Here's how the part is built. I have some questions about the finished solid (model axes, mm). A direction names the side the tool comes from. Round coordinates to 2 decimals unless told otherwise and drop trailing zeros. Order: outer loops, then holes, each group sorted by start corner. A loop starts at its lowest first (then second) coordinate and runs counter-clockwise, first axis right, second up. Notation, with made-up numbers: (54.25, 20.5) -> (75.25, 20.5) arc R33 cw to (75.25, 59.5) -> close; hole circle Ø11 at (11, -6.5). An arc over 180 degrees is marked (long way). Use a Markdown table: item, result. Add a question column.
(1) I want a section at B-B, the plane x = -7.5. Please give me the cut outline in (y, z), then the cut area to 3 significant figures.
(2) I'm going to push flat-ended pins straight in: P1, Ø2.5, axis at x = -27, y = 0, coming from the +Z side; P2, Ø1.3, axis at x = 27, y = 0, coming from the -Z side; P3, Ø0.5, axis at y = -1.5, z = 0.5, coming from the -X side. Where does each tip first touch, or does it pass through?
(3) I want a section at C-C, the plane z = 0.6. Please give me the cut outline in (x, y).
(4) I want a section at A-A, the plane y = 0. Please give me the cut outline in (x, z), then the cut area to 3 significant figures.
(5) Thinking about a two-plate mould opening in Y: for faces 1 (the face through (-0.6, 4.05, 0.5)), 2 (the face through (-29.95, 0.13, 0.49)), 3 (the face through (0.3, 5.95, 0.5)), 4 (the face through (-26.237, 0.24, 0.507)), which applies, pulls with the +Y half, pulls with the -Y half, needs draft (parallel to the pull), parting line crosses it, or undercut?
(6) If I drill on probe 1 along Y at (x, z) = (-2.5, 0.9); probe 2 along X at (y, z) = (-0.25, 0.7); probe 3 along X at (y, z) = (0.5, 0.15), over which ranges is the centre line in solid material (lowest first)?
(7) On a 3-axis mill with a long thin cutter (end or side, diameter ignored), from which of +Z, -Z, +X, -X, +Y, -Y can I reach the whole of each face in a straight line? I mean faces 5 (the face through (-0.6, -4.15, 0.5)), 6 (the face through (0, 5, 1)). Say none if no direction works.
(8) I want a section at D-D, the plane x = 27. Please give me the cut outline in (y, z), then the cut area to 3 significant figures.
from build123d import *

# Parameters (mm, degrees)
BOSS_EXTRUDE2_DEPTH = 1
SKETCH4_R           = 0.8
CUT_EXTRUDE1_DEPTH  = 31.551677532
SKETCH5_W           = 15.2
SKETCH5_H           = 8.2
CUT_EXTRUDE2_DEPTH  = 31.551677532


with BuildPart() as part:
    # Sketch3 → Boss-Extrude2 (new body)
    with BuildSketch(Plane.XY):
        with BuildLine():
            Line((24, 5.95), (-24, 5.95))
            ThreePointArc((-24, 5.95), (-29.95, 0), (-24, -5.95))
            Line((-24, -5.95), (24, -5.95))
            ThreePointArc((24, -5.95), (29.95, 0), (24, 5.95))
        make_face()
    extrude(amount=BOSS_EXTRUDE2_DEPTH)

    # Sketch4 → Cut-Extrude1 (cut, through all)
    with BuildSketch(Plane.XY.offset(1)):
        with Locations((-27, 0)):
            Circle(SKETCH4_R)
        with Locations((27, 0)):
            Circle(SKETCH4_R)
    extrude(amount=-CUT_EXTRUDE1_DEPTH, mode=Mode.SUBTRACT)

    # Sketch5 → Cut-Extrude2 (cut, through all)
    with BuildSketch(Plane.XY.offset(1)):
        with Locations((-0.5, -0.05)):
            Rectangle(SKETCH5_W, SKETCH5_H)
    extrude(amount=-CUT_EXTRUDE2_DEPTH, mode=Mode.SUBTRACT)


solid = part.part
Taken from the geometry:
| question | item | result |
|---|---|---|
| 1 | outline | (-5.95, 0) -> (-4.15, 0) -> (-4.15, 1) -> (-5.95, 1) -> close; (4.05, 0) -> (5.95, 0) -> (5.95, 1) -> (4.05, 1) -> close |
| 1 | area | 3.70 mm2 |
| 2 | P1 | stops at z = 1 |
| 2 | P2 | passes through |
| 2 | P3 | stops at x = -29.82 |
| 3 | outline | (-24, -5.95) -> (24, -5.95) arc R5.95 ccw to (24, 5.95) -> (-24, 5.95) arc R5.95 ccw to start; hole circle Ø1.6 at (-27, 0); hole (-8.1, -4.15) -> (7.1, -4.15) -> (7.1, 4.05) -> (-8.1, 4.05) -> close; hole circle Ø1.6 at (27, 0) |
| 4 | outline | (-29.95, 0) -> (-27.8, 0) -> (-27.8, 1) -> (-29.95, 1) -> close; (-26.2, 0) -> (-8.1, 0) -> (-8.1, 1) -> (-26.2, 1) -> close; (7.1, 0) -> (26.2, 0) -> (26.2, 1) -> (7.1, 1) -> close; (27.8, 0) -> (29.95, 0) -> (29.95, 1) -> (27.8, 1) -> close |
| 4 | area | 41.5 mm2 |
| 5 | face 1 | undercut |
| 5 | face 2 | parting line crosses it |
| 5 | face 3 | pulls with the +Y half |
| 5 | face 4 | undercut |
| 6 | probe 1 | y = -5.95 to -4.15, 4.05 to 5.95 |
| 6 | probe 2 | x = -29.94 to -27.76, -26.24 to -8.1, 7.1 to 26.24, 27.76 to 29.94 |
| 6 | probe 3 | x = -29.93 to -27.62, -26.38 to -8.1, 7.1 to 26.38, 27.62 to 29.93 |
| 7 | face 5 | +Z, -Z |
| 7 | face 6 | +Z, +X, -X, +Y, -Y |
| 8 | outline | (-5.14, 0) -> (-0.8, 0) -> (-0.8, 1) -> (-5.14, 1) -> close; (0.8, 0) -> (5.14, 0) -> (5.14, 1) -> (0.8, 1) -> close |
| 8 | area | 8.68 mm2 |
